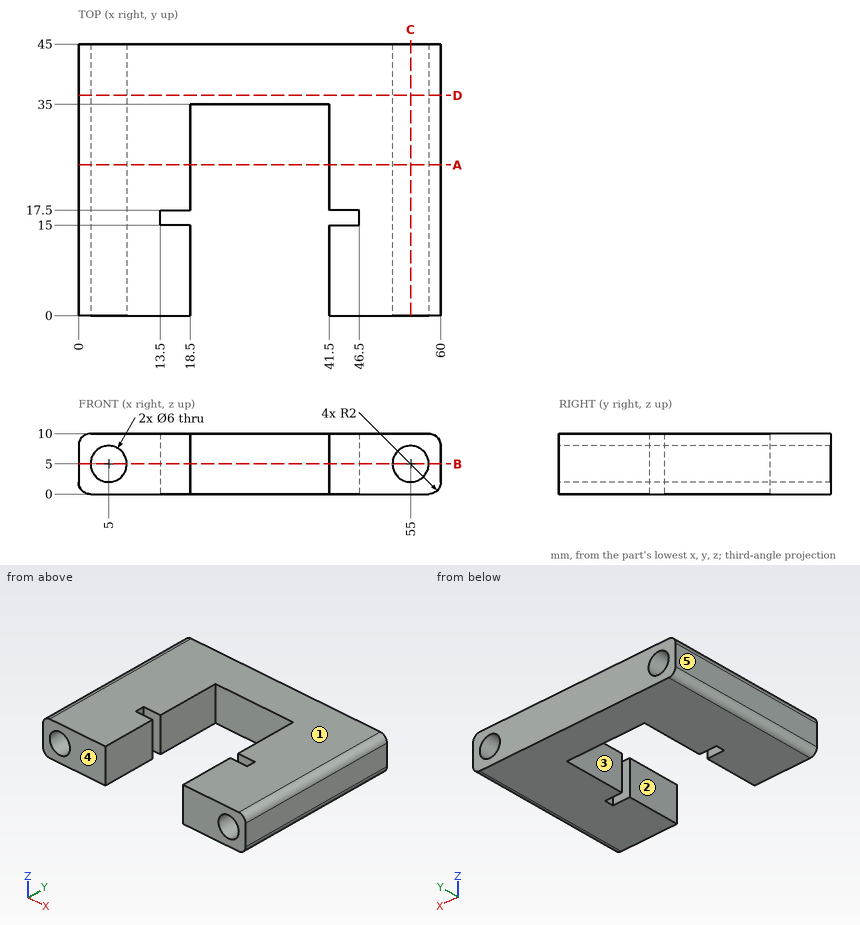
The drawing under review shows one solid part. Ordinate dimensions are in mm from its lowest x, y, z. A direction names the side the tool comes from. Give positions to 0.01 mm unless a question says otherwise; leave off trailing zeros. Write each loop counter-clockwise with the first axis right and the second up, starting at its lowest first coordinate (ties: lowest second). Pieces come first, ordered by that corner, then holes. Notation, with made-up numbers: (-8, 87) -> (30, 87) arc R15 cw to (30, 113) -> close; hole circle Ø9 at (-24, 58). An arc over 180 degrees is marked (long way). Use CSV: the item, a comma, the result in double quotes.
Q1. Mouldability with a two-part tool opening along X and no side actions: class the marked faces 3, 4 and 5 as pulls with the +X half, pulls with the -X half, needs draft (parallel to the pull), parting line crosses it, or undercut.
Conclusion:
face 3,"undercut"
face 4,"needs draft"
face 5,"pulls with the -X half"
Q2. For P1, Ø4, axis at x = 45, z = 4, coming from the -Y side; P2, Ø3, axis at x = 35.5, z = 6.5, coming from the -Y side, all flat-tipped, find the tip position at first contact; note any pin that passes through.
Conclusion:
P1,"y = 0"
P2,"y = 35"
Q3. Take a section at C-C, the plane x = 55. Write out the cut boundary in (y, z), then the cut area to 3 significant figures.
Conclusion:
outline,"(0, 0) -> (45, 0) -> (45, 2) -> (0, 2) -> close; (0, 8) -> (45, 8) -> (45, 10) -> (0, 10) -> close"
area,"180 mm2"
Q4. Tool access review of the marked faces 1 and 2: name each direction out of +Z, -Z, +X, -X, +Y, -Y from which nothing blocks a thin tool from reaching the whole face with its end or side.
Conclusion:
face 1,"+Z, +X, -X, +Y, -Y"
face 2,"+Z, -Z, -Y"
Q5. Take a section at A-A, the plane y = 25. Write out the cut boundary in (x, z), then the cut area to 3 significant figures.
Conclusion:
outline,"(0, 2) arc R2 ccw to (2, 0) -> (18.5, 0) -> (18.5, 10) -> (2, 10) arc R2 ccw to (0, 8) -> close; (41.5, 0) -> (58, 0) arc R2 ccw to (60, 2) -> (60, 8) arc R2 ccw to (58, 10) -> (41.5, 10) -> close; hole circle Ø6 at (5, 5); hole circle Ø6 at (55, 5)"
area,"310 mm2"
Q6. Take a section at D-D, the plane y = 36.5. Write out the cut boundary in (x, z).
Conclusion:
outline,"(0, 2) arc R2 ccw to (2, 0) -> (58, 0) arc R2 ccw to (60, 2) -> (60, 8) arc R2 ccw to (58, 10) -> (2, 10) arc R2 ccw to (0, 8) -> close; hole circle Ø6 at (5, 5); hole circle Ø6 at (55, 5)"
Q7. To check wall thickness, follow probe 1 along X at (y, z) = (12, 5); probe 2 along Z at (x, y) = (55, 30); probe 3 along Y at (x, z) = (15, 5). State the ranges of each line that lie inside material, in increasing order. Write a range as [from, to].
Conclusion:
probe 1,"[0, 2], [8, 18.5], [41.5, 52], [58, 60]"
probe 2,"[0, 2], [8, 10]"
probe 3,"[0, 15], [17.5, 45]"
Q8. Take a section at B-B, the plane z = 5. Write out the cut boundary in (x, y), then the cut area to 3 significant figures.
Conclusion:
outline,"(0, 0) -> (2, 0) -> (2, 45) -> (0, 45) -> close; (8, 0) -> (18.5, 0) -> (18.5, 15) -> (13.5, 15) -> (13.5, 17.5) -> (18.5, 17.5) -> (18.5, 35) -> (41.5, 35) -> (41.5, 17.5) -> (46.5, 17.5) -> (46.5, 15) -> (41.5, 15) -> (41.5, 0) -> (52, 0) -> (52, 45) -> (8, 45) -> close; (58, 0) -> (60, 0) -> (60, 45) -> (58, 45) -> close"
area,"1,330 mm2"
